Source: CAD feature listing. Evaluate the final solid. Frame: model axes, mm. Face numbers are marked on the shaded views. A direction names the side the tool comes from. Give positions to 0.01 mm unless a question says otherwise; leave off trailing zeros. Loops run counter-clockwise (first coordinate to the right, second up) from the corner with the lowest first, then second, coordinate; pieces in that order, holes last. Notation, with made-up numbers: (34.5, -24) - (85.5, -24) arc R23 cw to (85.5, -14) - close; hole circle Ø5 at (79, 85.5). An arc over 180 degrees is marked (long way). Write each question's results on one line, items separated by ' | '. Start each with the question number.
(1) Material intervals for line 1 along X through (y, z) = (5.4, 0); line 2 along Z through (x, y) = (9, 0); line 3 along Z through (x, y) = (40, -0.25), sorted ascending. Write a range as [from, to].
(2) Cut plane A-A on x = 31.5. Return the cut outline in (y, z).
(3) Pull-direction query (Y, two-part tool) for the marked faces 5, 6, 7 and 8; classes: pulls with the +Y half, pulls with the -Y half, needs draft (parallel to the pull), parting line crosses it, or undercut.
(4) Reachability of the marked faces 1, 2, 3 and 4 from +Z, -Z, +X, -X, +Y, -Y: full face, straight path, thin tool, end or side. Return the list, or none.
(5) Cut plane B-B on z = 3. Return the cut outline in (x, y), then the cut area to 3 significant figures.
(6) Cut plane D-D on z = -4.5. Return the cut outline in (x, y).
(7) Contact query for flat-ended pins moving along their axis: pin 1 (4 mm diameter, centred on x = 31, z = 5.5, fed in from -Y); pin 2 (3 mm diameter, centred on x = 24, z = -2, fed in from -Y); pin 3 (2.5 mm diameter, centred on y = 1.5, z = 1.5, fed in from +X). Output: stop coordinate, or through.
(8) Cut plane C-C on y = 7. Return the cut outline in (x, z), then the cut area to 3 significant figures.
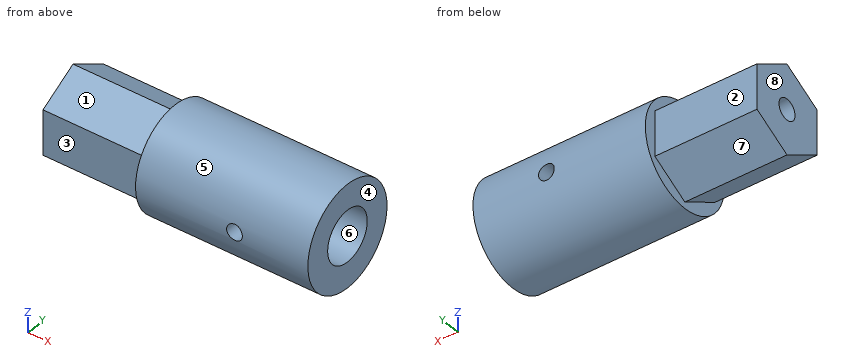
Autodesk Inventor part; units mm, degrees
ref_plane "РабПлоскость1" through (0, 9, 0) normal (0, 1, 0) x (-1, 0, 0)
ref_plane "YZ Plane" through (0, 0, 0) normal (1, 0, 0) x (0, 1, 0)
ref_plane "XY Plane" through (0, 0, 0) normal (0, 0, 1) x (1, 0, 0)
sketch "Эскиз1" plane through (0, 0, 0) normal (1, 0, 0) x (0, 1, 0)
  line L0 (6.0622, 3.5) -> (6.0622, -3.5)
  line L1 (6.0622, -3.5) -> (0, -7)
  line L2 (0, -7) -> (-6.0622, -3.5)
  line L3 (-6.0622, -3.5) -> (-6.0622, 3.5)
  line L4 (-6.0622, 3.5) -> (0, 7)
  line L5 (0, 7) -> (6.0622, 3.5)
  circle A0 centre (0, 0) radius 7 construction
  dimension "d0" = 14
extrude "Выдавливание1" add sketch "Эскиз1" along normal blind 25
sketch "Эскиз2" plane through (25, 0, 0) normal (1, 0, 0) x (0, 0, -1)
  circle A0 centre (0, 0) radius 8
  circle A1 centre (0, 0) radius 4
  dimension "d3" = 16
  dimension "d6" = 8
extrude "Выдавливание2" add sketch "Эскиз2" along normal blind 18 and the other way blind 9
ref_plane "РабПлоскость1" through (0, 9, 0) normal (0, 1, 0) x (-1, 0, 0)
sketch "Эскиз3" plane through (0, 9, 0) normal (0, 1, 0) x (-1, 0, 0)
  line L0 (-43, 8) -> (-43, -8)
  point P0 (0, 0)
  point P1 (-31.5, 0)
  dimension "d16" = 11.5
hole "Отверстие1" at (31.5, 9, 0) direction (0, -1, 0) diameter 2.459 end through all
sketch "Эскиз4" plane through (0, 0, 0) normal (-1, 0, 0) x (0, 0, 1)
  point P0 (0, 0)
  point P1 (0, 0)
hole "Отверстие2" at (0, 0, 0) direction (1, 0, 0) diameter 3.242 depth 11.8 tip angle 118
properties part number "переходная втулка"
Ans:
1) line 1: [0, 30.27], [32.73, 43] | line 2: [-7, -1.62], [1.62, 7] | line 3: [-8, -3.99], [3.99, 8]
2) outline: (-7.9, -1.23) arc R8 ccw to (7.9, -1.23) - (3.81, -1.23) arc R4 cw to (-3.81, -1.23) - close; (-7.9, 1.23) - (-3.81, 1.23) arc R4 cw to (3.81, 1.23) - (7.9, 1.23) arc R8 ccw to start
3) face 5: parting line crosses it | face 6: undercut | face 7: pulls with the +Y half | face 8: needs draft
4) face 1: +Z, -X, -Y | face 2: +Z, -Z, -X, +Y | face 3: +Z, -Z, -X, -Y | face 4: +Z, -Z, +X, +Y, -Y
5) outline: (0, -6.06) - (16, -6.06) - (16, -7.42) - (43, -7.42) - (43, -2.65) - (25, -2.65) - (25, 2.65) - (43, 2.65) - (43, 7.42) - (16, 7.42) - (16, 6.06) - (0, 6.06) - close | area: 499 mm^2
6) outline: (0, -4.33) - (16, -4.33) - (16, -6.61) - (43, -6.61) - (43, 6.61) - (16, 6.61) - (16, 4.33) - (0, 4.33) - close
7) pin 1: y = -7.19 | pin 2: y = -7.98 | pin 3: x = 25
8) outline: (16, -3.87) - (43, -3.87) - (43, 3.87) - (16, 3.87) - close; hole circle Ø2.46 at (31.5, 0) | area: 204 mm^2
